For this review, take the finished solid that the model builds, in its own axes (mm). A direction names the side the tool comes from. Give positions to 0.01 mm unless a question says otherwise; leave off trailing zeros. Write each loop counter-clockwise with the first axis right and the second up, starting at its lowest first coordinate (ties: lowest second). Pieces come first, ordered by that corner, then holes.
from build123d import *

# Parameters (mm, degrees)
SKETCH1_R           = 50
BOSS_EXTRUDE1_DEPTH = 40
CIRPATTERN1_COUNT   = 10
FILLET2_R           = 3
SKETCH9_R           = 5
CUT_EXTRUDE2_DEPTH  = 90.970332195
SKETCH10_R          = 47
SKETCH10_R_2        = 30
CUT_EXTRUDE3_DEPTH  = 15
CUT_EXTRUDE4_START  = 5
CUT_EXTRUDE4_DEPTH  = 5
CIRPATTERN2_COUNT   = 10


with BuildPart() as part:
    # Sketch1 → Boss-Extrude1 (new body)
    with BuildSketch(Plane(origin=(0, 0, 0), x_dir=(1, 0, 0), z_dir=(0, 1, 0))):
        with Locations(Location((0, 0, 0), (0, 0, 270))):
            Circle(SKETCH1_R)
    extrude(amount=BOSS_EXTRUDE1_DEPTH)

    # Sketch5 → CSK for M5 Countersunk Flat Head Screw1 (revolve, cut)
    with BuildSketch(Plane(origin=(-37.983874715, 40, -1.585807891), x_dir=(0, 0, 1), z_dir=(1, 0, 0))):
        Polygon((0, 0), (0, 16.652366702), (2.75, 15), (2.75, 2.45), (5.2, 0), align=None)
    csk_for_m5_countersunk_flat_head_screw1 = revolve(axis=Axis((-37.983874715, 46.35, -1.585807891), (0, -1, 0)), mode=Mode.SUBTRACT)

    # CirPattern1: CSK for M5 Countersunk Flat Head Screw1 ×10 about axis
    cirpattern1_axis = Axis((0, 0, 0), (0, 1, 0))
    for i in range(1, CIRPATTERN1_COUNT):
        add(csk_for_m5_countersunk_flat_head_screw1.rotate(cirpattern1_axis, i * 360 / CIRPATTERN1_COUNT), mode=Mode.SUBTRACT)

    # Fillet2
    fillet2_edges = [part.edges().sort_by_distance(p)[0] for p in [
        (0, 40, -50),
    ]]
    fillet(fillet2_edges, radius=FILLET2_R)

    # Sketch8 → Revolve2 (revolve)
    with BuildSketch(Plane(origin=(0, 0, 0), x_dir=(0, 0, -1), z_dir=(1, 0, 0))):
        with BuildLine():
            Line((-50, 0), (0, 0))
            Line((0, 0), (0, -15.629674134))
            ThreePointArc((0, -15.629674134), (-25.977086096, -10.940577527), (-50, 0))
        make_face()
    revolve(axis=Axis((0, 0, 0), (0, -1, 0)))

    # Sketch9 → Cut-Extrude2 (cut, through all)
    with BuildSketch(Plane(origin=(0, 40, 0), x_dir=(1, 0, 0), z_dir=(0, 1, 0))):
        with Locations(Location((0, 0, 0), (0, 0, 270))):
            Circle(SKETCH9_R)
    extrude(amount=-CUT_EXTRUDE2_DEPTH, mode=Mode.SUBTRACT)

    # Sketch10 → Cut-Extrude3 (cut)
    with BuildSketch(Plane(origin=(0, 25, 0), x_dir=(1, 0, 0), z_dir=(0, 1, 0))):
        with Locations(Location((0, 0, 0), (0, 0, 270))):
            Circle(SKETCH10_R)
        with Locations(Location((0, 0, 0), (0, 0, 270))):
            Circle(SKETCH10_R_2, mode=Mode.SUBTRACT)
    extrude(amount=-CUT_EXTRUDE3_DEPTH, mode=Mode.SUBTRACT)

    # Sketch15 → Cut-Extrude4 (cut)
    with BuildSketch(Plane(origin=(0, 10, 0), x_dir=(1, 0, 0), z_dir=(0, 1, 0)).offset(CUT_EXTRUDE4_START)):
        with BuildLine():
            Line((4.527076374, -2.122635039), (25.067176095, -16.504967699))
            ThreePointArc((25.067176095, -16.504967699), (24.302227971, -17.611899153), (23.488435591, -18.683433026))
            Line((23.488435591, -18.683433026), (3.470823887, -3.599080653))
            ThreePointArc((3.470823887, -3.599080653), (4.066518789, -2.909196615), (4.527076374, -2.122635039))
        make_face()
    cut_extrude4 = extrude(amount=-CUT_EXTRUDE4_DEPTH, mode=Mode.SUBTRACT)

    # CirPattern2: Cut-Extrude4 ×10 about axis
    cirpattern2_axis = Axis((0, 0, 0), (0, 1, 0))
    for i in range(1, CIRPATTERN2_COUNT):
        add(cut_extrude4.rotate(cirpattern2_axis, i * 360 / CIRPATTERN2_COUNT), mode=Mode.SUBTRACT)


solid = part.part
(1) We need section B-B (y = 4). Write out the cut boundary in (x, z).
(2) Tool access review of faces 3 (the cylindrical face through (-3, 13, -4)), 4 (the flat face through (19, 15, 0)), 5 (the cylindrical face through (-34.357, 31.363, 20.496)): name each direction out of +Z, -Z, +X, -X, +Y, -Y from which nothing blocks a thin tool from reaching the whole face with its end or side.
(3) For L1, parallel to X at y = 32.5, z = 22.5; L2, parallel to X at y = 14, z = 0; L3, parallel to X at y = 22.5, z = 18.5, list the stretches that pass through material, from the lowest coordinate up.
(4) We need section A-A (y = 27.5). Count the separate pieces of the cut face and the enclosed holes in it, and give its area (3 significant figures).
(5) Clearance check with flat-ended pins moving along their axes: pin 1 Ø3.5 at (x, z) = (29.8, 23.61) entering from +Y; pin 2 Ø5 at (x, z) = (7.5, 15) entering from -Y; pin 3 Ø8 at (x, z) = (4, -13) entering from -Y. State where each tip first meets the part, or that it passes through.
(6) The part is to be moulded in two halves that separate along Z. For faces 1 (the flat face through (-14.65, 12.54, -9.21)), 2 (the flat face through (13.29, 12.54, -11.09)), say which applies: +Z half, -Z half, draft (parallel to the pull), parting line (faces both ways), or undercut.
The answers:
1. outline: circle Ø100 at (0, 0); hole circle Ø10 at (0, 0)
2. face 3: +Y, -Y
2. face 4: none
2. face 5: +Y
3. L1: x = -44.65 to -33.99, -29.33 to 27.28, 32.31 to 44.65
3. L2: x = -50 to -47, 47 to 50
3. L3: x = -46.45 to -43.21, -23.62 to 23.62, 43.21 to 46.45
4. separate pieces: 1
4. enclosed holes: 11
4. area: 7,540 mm2
5. pin 1: stops at y = 10
5. pin 2: stops at y = -13.88
5. pin 3: stops at y = -14.67
6. face 1: undercut
6. face 2: undercut
